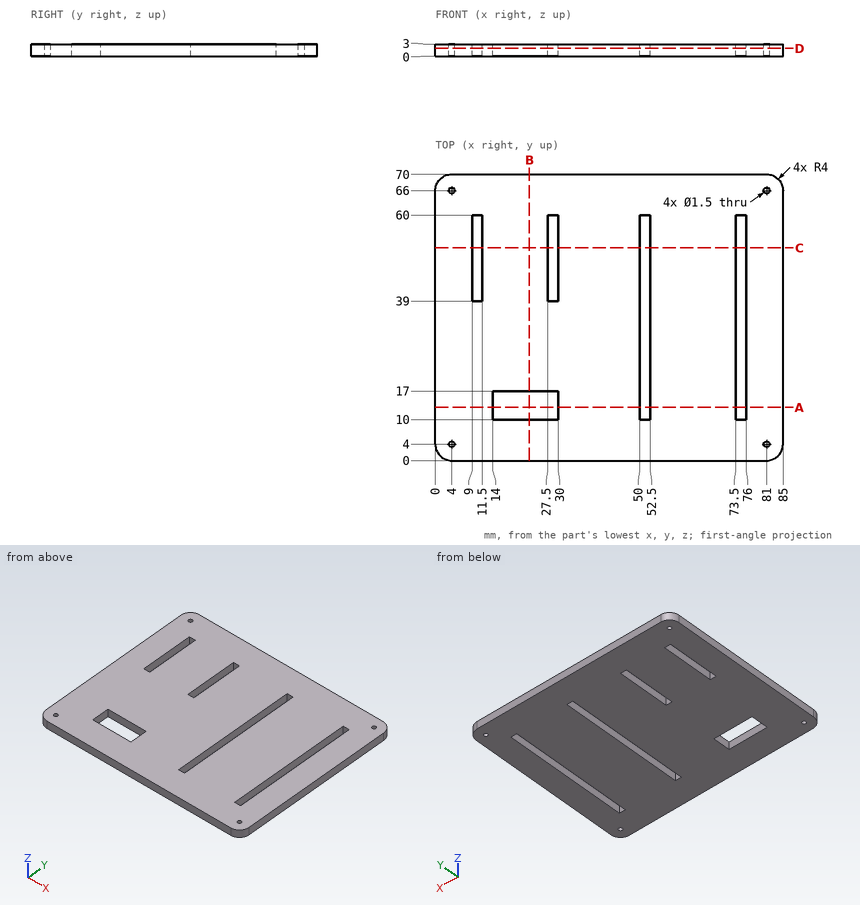
Geometry: see drawing. Coordinates: mm, zero at the bounding-box minimum. Give positions to 0.01 mm unless a question says otherwise; leave off trailing zeros. Write each loop counter-clockwise with the first axis right and the second up, starting at its lowest first coordinate (ties: lowest second). Pieces come first, ordered by that corner, then holes. Notation, with made-up numbers: (31.5, 60.25) -> (77.5, 60.25) arc R5 ccw to (77.5, 67.25) -> close; hole circle Ø2 at (28, 28.25). An arc over 180 degrees is marked (long way). Use one line per item in the form item = value. Start each with the question number.
1) Section query C-C on y = 52. Return the cut outline in (x, z), then the cut area to 3 significant figures.
2) Section query D-D on z = 1.95. Count the separate pieces of the cut face and the enclosed holes in it, then the cut area to 3 significant figures.
3) Ray query, probe 1 along Y at (x, z) = (81, 1.1); probe 2 along X at (y, z) = (24.5, 0.2); probe 3 along X at (y, z) = (66, 1.15). Return the intervals inside material, ascending. Write a range as from..to.
4) Pin query (flat end, axial travel): pin 1 (1.4 mm diameter, centred on x = 4, y = 66, fed in from +Z). Return the tip coordinate at first contact, or that it passes through.
5) Section query A-A on y = 13. Return the cut outline in (x, z), then the cut area to 3 significant figures.
6) Section query B-B on x = 23. Return the cut outline in (y, z).
Outcome:
q1.outline = (0, 0) -> (9, 0) -> (9, 3) -> (0, 3) -> close; (11.5, 0) -> (27.5, 0) -> (27.5, 3) -> (11.5, 3) -> close; (30, 0) -> (50, 0) -> (50, 3) -> (30, 3) -> close; (52.5, 0) -> (73.5, 0) -> (73.5, 3) -> (52.5, 3) -> close; (76, 0) -> (85, 0) -> (85, 3) -> (76, 3) -> close
q1.area = 225 mm^2
q2.separate_pieces = 1
q2.enclosed_holes = 9
q2.area = 5,460 mm^2
q3.probe_1 = 0..3.25, 4.75..65.25, 66.75..70
q3.probe_2 = 0..50, 52.5..73.5, 76..85
q3.probe_3 = 0..3.25, 4.75..80.25, 81.75..85
q4.pin_1 = through
q5.outline = (0, 0) -> (14, 0) -> (14, 3) -> (0, 3) -> close; (30, 0) -> (50, 0) -> (50, 3) -> (30, 3) -> close; (52.5, 0) -> (73.5, 0) -> (73.5, 3) -> (52.5, 3) -> close; (76, 0) -> (85, 0) -> (85, 3) -> (76, 3) -> close
q5.area = 192 mm^2
q6.outline = (0, 0) -> (10, 0) -> (10, 3) -> (0, 3) -> close; (17, 0) -> (70, 0) -> (70, 3) -> (17, 3) -> close
